Can you work these out from the model? Positions are in its coordinate system, mm. Round coordinates to 2 decimals unless told otherwise and drop trailing zeros. Answer as CSV lines item,"result".
```python
from build123d import *

# Parameters (mm, degrees)
SKETCH1_R           = 0.5
SKETCH1_R_2         = 1.004584714
SKETCH1_R_3         = 1
BOSS_EXTRUDE4_DEPTH = 2


with BuildPart() as part:
    # Sketch1 → Boss-Extrude4 (new body)
    with BuildSketch(Plane.XY):
        with BuildLine():
            Line((0, 6.796629536), (0, 23.203370382))
            add(Edge.make_bspline(
                [(0, 23.203370382), (18.824108825, 19.022876047), (31.816291347, 34.013726018)],
                knots=[0, 0, 0, 1, 1, 1], degree=2))
            Line((31.816291347, 34.013726018), (31.816291347, -2.297085155))
            add(Edge.make_bspline(
                [(0, 6.796629536), (18.47321861, 12.396952678), (31.816291347, -2.297085155)],
                knots=[0, 0, 0, 1, 1, 1], degree=2))
        make_face()
        with Locations((7.382147853, 19.853448191)):
            Circle(SKETCH1_R, mode=Mode.SUBTRACT)
        with Locations((7.382147853, 9.889606803)):
            Circle(SKETCH1_R, mode=Mode.SUBTRACT)
        with Locations((7.382147853, 14.871527497)):
            Circle(SKETCH1_R, mode=Mode.SUBTRACT)
        with Locations((30.227051082, 29.675836966)):
            Circle(SKETCH1_R_2, mode=Mode.SUBTRACT)
        with Locations((30.230334009, 2.675837166)):
            Circle(SKETCH1_R_3, mode=Mode.SUBTRACT)
    extrude(amount=BOSS_EXTRUDE4_DEPTH)


solid = part.part
```
Q1. I'm going to push flat-ended pins straight in: pin 1 Ø1.8 at (x, y) = (30.23, 2.68) entering from +Z; pin 2 Ø8 at (x, y) = (7, 23.5) entering from -Z. Where does each tip first touch, or does it pass through?
Checks:
pin 1,"through"
pin 2,"z = 0"
Q2. We'd pull the mould along X, two halves only. Please class faces 1 (the cylindrical face through (7.651, 15.293, 0.986)), 2 (the flat face through (31.816, 16, 1)), 3 (the flat face through (0, 15, 1)): pulls with the +X half, pulls with the -X half, needs draft (parallel to the pull), parting line crosses it, or undercut.
Checks:
face 1,"undercut"
face 2,"pulls with the +X half"
face 3,"pulls with the -X half"
Q3. Imagine slicing it at A-A (z = 1.1). Count the separate pieces of the cut face and the enclosed holes in it, then the cut area to 3 significant figures.
Checks:
separate pieces,"1"
enclosed holes,"5"
area,"602 mm²"
Q4. If I drill on line 1 along X through (y, z) = (32.5, 0.8); line 2 along Y through (x, z) = (10, 0.3); line 3 along Y through (x, z) = (15, 1.5), over which ranges is the centre line in solid material (lowest first)? Write a range as [from, to].
Checks:
line 1,"[30.44, 31.82]"
line 2,"[8.34, 22.36]"
line 3,"[7.85, 23.13]"
